from build123d import *

# Parameters (mm, degrees)
PAD_DEPTH       = 15
SKETCH002_R     = 20
POCKET_DEPTH    = 3
POCKET001_DEPTH = 7
FILLET_R        = 2
FILLET001_R     = 2


with BuildPart() as part:
    # Sketch → Pad (new body)
    with BuildSketch(Plane.XY):
        Polygon((0, 30), (-25.980762, 15), (-25.980762, -15), (0, -30), (25.980762, -15), (25.980762, 15), align=None)
    extrude(amount=PAD_DEPTH)

    # Sketch002 (on Face8 of Pad) → Pocket (cut)
    with BuildSketch(Plane.XY.offset(15)):
        Circle(SKETCH002_R)
    extrude(amount=-POCKET_DEPTH, mode=Mode.SUBTRACT)

    # Sketch003 (on Face10 of Pocket) → Pocket001 (cut)
    with BuildSketch(Plane.XY.offset(12)):
        Polygon((0, 9.814955), (-8.5, 4.907477), (-8.5, -4.907477), (0, -9.814955), (8.5, -4.907477), (8.5, 4.907477), align=None)
    extrude(amount=-POCKET001_DEPTH, mode=Mode.SUBTRACT)

    # Fillet
    fillet_edges = [part.edges().sort_by_distance(p)[0] for p in [
        (25.980762, 0, 15),
        (12.990381, -22.5, 15),
        (-12.990381, -22.5, 15),
        (-25.980762, 0, 15),
        (-12.990381, 22.5, 15),
        (12.990381, 22.5, 15),
        (25.980762, 0, 0),
        (12.990381, -22.5, 0),
        (-12.990381, -22.5, 0),
        (12.990381, 22.5, 0),
        (-12.990381, 22.5, 0),
        (-25.980762, 0, 0),
    ]]
    fillet(fillet_edges, radius=FILLET_R)

    # Fillet001
    fillet001_edges = [part.edges().sort_by_distance(p)[0] for p in [
        (0, 30, 7.5),
        (-25.980762, 15, 7.5),
        (-25.980762, -15, 7.5),
        (0, -30, 7.5),
        (25.980762, -15, 7.5),
        (25.980762, 15, 7.5),
    ]]
    fillet(fillet001_edges, radius=FILLET001_R)


solid = part.part
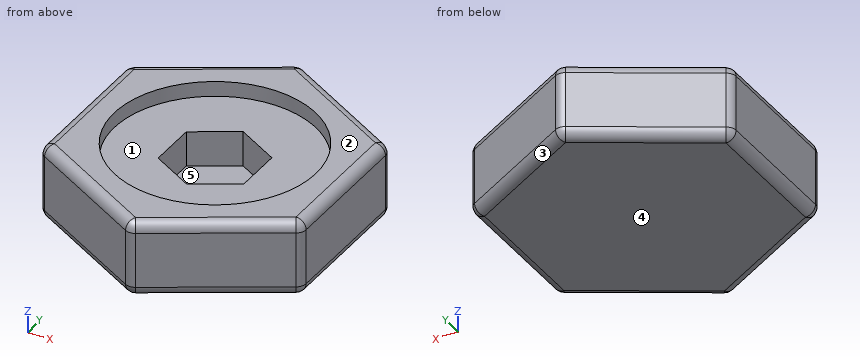
For this review, take the finished solid that the model builds, in its own axes (mm). Face numbers are marked on the shaded views. A direction names the side the tool comes from. Round coordinates to 2 decimals unless told otherwise and drop trailing zeros. Order: outer loops, then holes, each group sorted by start corner. A loop starts at its lowest first (then second) coordinate and runs counter-clockwise, first axis right, second up. Notation, with made-up numbers: (32, -27.5) -> (78, -27.5) arc R3 cw to (78, -23.5) -> close; hole circle Ø10 at (-14, -14). An arc over 180 degrees is marked (long way). Put each result on its own line as item: value.
Q1. Add section C-C on z = 3.25. Write out the cut boundary in (x, y), plus the area to 3 significant figures.
Check result:
outline: (-25.98, -13.85) arc R2 ccw to (-24.98, -15.58) -> (-1, -29.42) arc R2 ccw to (1, -29.42) -> (24.98, -15.58) arc R2 ccw to (25.98, -13.85) -> (25.98, 13.85) arc R2 ccw to (24.98, 15.58) -> (1, 29.42) arc R2 ccw to (-1, 29.42) -> (-24.98, 15.58) arc R2 ccw to (-25.98, 13.85) -> close
area: 2,340 mm2
Q2. Mouldability with a two-part tool opening along X and no side actions: class the marked faces 3, 4 and 5 as pulls with the +X half, pulls with the -X half, needs draft (parallel to the pull), parting line crosses it, or undercut.
Check result:
face 3: pulls with the +X half
face 4: needs draft
face 5: undercut
Q3. Add section D-D on y = -11.5. Write out the cut boundary in (x, z), plus the area to 3 significant figures.
Check result:
outline: (-25.98, 2) arc R2 ccw to (-23.98, 0) -> (23.98, 0) arc R2 ccw to (25.98, 2) -> (25.98, 13) arc R2 ccw to (23.98, 15) -> (16.36, 15) -> (16.36, 12) -> (-16.36, 12) -> (-16.36, 15) -> (-23.98, 15) arc R2 ccw to (-25.98, 13) -> close
area: 678 mm2
Q4. Add section A-A on z = 9. Write out the cut boundary in (x, y), plus the area to 3 significant figures.
Check result:
outline: (-25.98, -13.85) arc R2 ccw to (-24.98, -15.58) -> (-1, -29.42) arc R2 ccw to (1, -29.42) -> (24.98, -15.58) arc R2 ccw to (25.98, -13.85) -> (25.98, 13.85) arc R2 ccw to (24.98, 15.58) -> (1, 29.42) arc R2 ccw to (-1, 29.42) -> (-24.98, 15.58) arc R2 ccw to (-25.98, 13.85) -> close; hole (-8.5, -4.91) -> (0, -9.81) -> (8.5, -4.91) -> (8.5, 4.91) -> (0, 9.81) -> (-8.5, 4.91) -> close
area: 2,090 mm2
Q5. For probe 1 along Y at (x, z) = (0, 13.15); probe 2 along X at (y, z) = (4, 8.5); probe 3 along X at (y, z) = (-21, 13), list the stretches that pass through material, from the lowest coordinate up. Write a range as [from, to].
Check result:
probe 1: [-29.68, -20], [20, 29.68]
probe 2: [-25.98, -8.5], [8.5, 25.98]
probe 3: [-15.59, 15.59]
Q6. Machinability: for the marked faces 1 and 2, which of the approach directions +Z, -Z, +X, -X, +Y, -Y give a long, thin tool a straight path to every point of the face, cutting with its end or side? Answer none if there is none.
Check result:
face 1: +Z
face 2: +Z, +X, -X, +Y, -Y
Q7. Insertion check: pin 1 Ø3 at (x, z) = (-4.5, 7.5) entering from -Y; pin 2 Ø13.5 at (x, y) = (0.5, 1.5) entering from +Z; pin 3 Ø8 at (y, z) = (17, 10.5) entering from +X; pin 4 Ø3 at (x, z) = (-18.5, 5.5) entering from +Y. Each pin has a flat end and moves straight along its axis. Give the tip position at first contact, or say it passes through.
Check result:
pin 1: y = -28.27
pin 2: z = 5
pin 3: x = 25.98
pin 4: y = 20.19
Q8. Add section B-B on y = 0. Write out the cut boundary in (x, z).
Check result:
outline: (-25.98, 2) arc R2 ccw to (-23.98, 0) -> (23.98, 0) arc R2 ccw to (25.98, 2) -> (25.98, 13) arc R2 ccw to (23.98, 15) -> (20, 15) -> (20, 12) -> (8.5, 12) -> (8.5, 5) -> (-8.5, 5) -> (-8.5, 12) -> (-20, 12) -> (-20, 15) -> (-23.98, 15) arc R2 ccw to (-25.98, 13) -> close
